Build history of the part. All positions in model axes, mm. A direction names the side the tool comes from. Coordinates: 2 decimals unless noted, no trailing zeros. Order: outer loops, then holes, each group sorted by start corner. A loop starts at its lowest first (then second) coordinate and runs counter-clockwise, first axis right, second up. Notation, with made-up numbers: (51, -21.5) - (102, -21.5) arc R22 ccw to (102, -2.5) - close; hole circle Ø10 at (80, 11.5). An arc over 180 degrees is marked (long way). Return JSON: item names as keys, results as strings.
Autodesk Inventor part; units mm, degrees
ref_plane "YZ Plane" through (0, 0, 0) normal (1, 0, 0) x (0, 1, 0)
ref_plane "XZ Plane" through (0, 0, 0) normal (0, 1, 0) x (-1, 0, 0)
ref_plane "XY Plane" through (0, 0, 0) normal (0, 0, 1) x (1, 0, 0)
sketch "Эскиз1" plane through (0, 0, 0) normal (0, 1, 0) x (-1, 0, 0)
  line L0 (4, -4) -> (-4, -4)
  line L1 (-4, -4) -> (-4, 4)
  line L2 (-4, 4) -> (4, 4)
  line L3 (4, 4) -> (4, -4)
  circle A0 centre (0, 0) radius 10
  point P0 (-4, 0)
  point P1 (0, -4)
  dimension "d0" = 8
  dimension "d1" = 20
extrude "Выдавливание1" add sketch "Эскиз1" along normal mid plane 4
thread "Резьба1"
properties part number "80. Стопор предохранителя"
1. Probe L1, parallel to Z at x = -1, y = -1.4; L2, parallel to X at y = 1.3, z = 3.75; L3, parallel to Z at x = -0.25, y = -0.8. List the from-to ranges inside material, lowest first.
Check values:
{"L1": "-9.95 to -4, 4 to 9.95", "L2": "-9.27 to -4, 4 to 9.27", "L3": "-10 to -4, 4 to 10"}
2. Cut at B-B on x = 0. Give the cut face in (y, z).
Check values:
{"outline": "(-2, -10) - (2, -10) - (2, -4) - (-2, -4) - close; (-2, 4) - (2, 4) - (2, 10) - (-2, 10) - close"}
3. Cut at A-A on z = 0. Give the cut face in (x, y).
Check values:
{"outline": "(-10, -2) - (-4, -2) - (-4, 2) - (-10, 2) - close; (4, -2) - (10, -2) - (10, 2) - (4, 2) - close"}
4. Mould opens along Z. For faces 1 (the cylindrical face through (2.17, -0.03, 9.76)), 2 (the flat face through (4, 0, 0)), 3 (the flat face through (-4.3, -2, 0.1)) say: pulls with the +Z half, pulls with the -Z half, needs draft (parallel to the pull), parting line crosses it, or undercut.
Check values:
{"face 1": "parting line crosses it", "face 2": "undercut", "face 3": "needs draft"}
5. Drop a flat-ended pin along its axis: pin 1 (1.2 mm diameter, centred on y = -0.5, z = 1.5, fed in from +X). Give the stop position or say it passes through.
Check values:
{"pin 1": "x = 9.96"}
6. Tool access for faces 4 (the flat face through (-4.3, 2, 0.1)), 5 (the flat face through (0, 0, -4)): list every direction of +Z, -Z, +X, -X, +Y, -Y with a clear straight run to the whole face (end or side of a thin tool).
Check values:
{"face 4": "+Z, -Z, +X, -X, +Y", "face 5": "+Y, -Y"}
7. Cut at C-C on y = 1.3. Give the cut face in (x, z).
Check values:
{"outline": "circle Ø20 at (0, 0); hole (-4, -4) - (4, -4) - (4, 4) - (-4, 4) - close"}
8. Cut at D-D on x = 6.5. Give the cut face in (y, z).
Check values:
{"outline": "(-2, -7.6) - (2, -7.6) - (2, 7.6) - (-2, 7.6) - close"}
